Autodesk Inventor part; units mm, degrees
ref_plane "YZ Plane" through (0, 0, 0) normal (1, 0, 0) x (0, 1, 0)
ref_plane "XZ Plane" through (0, 0, 0) normal (0, 1, 0) x (-1, 0, 0)
ref_plane "XY Plane" through (0, 0, 0) normal (0, 0, 1) x (1, 0, 0)
sketch "Sketch1" plane through (0, 0, 0) normal (0, 1, 0) x (-1, 0, 0)
  circle A0 centre (0, 0) radius 25
  dimension "d0" = 50
extrude "Extrusion1" add sketch "Sketch1" against normal blind 15
sketch "Sketch3" plane through (0, 0, 0) normal (0, 1, 0) x (-1, 0, 0)
  circle A0 centre (0, 0) radius 15
  dimension "d3" = 30
extrude "Extrusion2" cut sketch "Sketch3" against normal through all
sketch "Sketch4" plane through (0, 0, 0) normal (0, 1, 0) x (-1, 0, 0)
  circle A0 centre (0, 0) radius 20
  dimension "d6" = 40
extrude "Extrusion3" cut sketch "Sketch4" against normal blind 12
properties part number "Седло для подшипника"
Geometry check sheet. Reference: the model listing, model coordinates, mm. Round coordinates to 2 decimals unless told otherwise and drop trailing zeros. Loops run counter-clockwise (first coordinate to the right, second up) from the corner with the lowest first, then second, coordinate; pieces in that order, holes last. Notation, with made-up numbers: (63, 37.25) - (102, 37.25) arc R17 ccw to (102, 47.25) - close; hole circle Ø11 at (51, -27). An arc over 180 degrees is marked (long way). Write each question's results on one line, items separated by ' | '. Start each with the question number.
Q1. Release check for a two-part mould opening along X. For faces 1 (the flat face through (-3, -12, 15)), 2 (the cylindrical face through (-23.846, -7.395, 7.509)), 3 (the flat face through (11, 0, 17)), 4 (the cylindrical face through (4.336, -5.916, -19.524)) record: +X half, -X half, draft (parallel to the pull), parting line (faces both ways), or undercut.
Q2. Cross-section at C-C on y = -10. Enter the section's corners in (x, z), and give its area (3 significant figures).
Q3. Cross-section at B-B on z = 0. Enter the section's corners in (x, y), and give its area (3 significant figures).
Q4. Cross-section at A-A on x = 0. Enter the section's corners in (y, z), and give its area (3 significant figures).
Q5. Thickness scan on line 1 (Z direction, x = 0, y = -13.3); line 2 (Z direction, x = 0, y = -3); line 3 (Y direction, x = -3.5, z = -19.5). Record the ranges inside material, lowest first. Write a range as [from, to].
Q6. Gauge pin test, flat ends, axial feed: P1, Ø2, axis at x = 17.5, z = -3, coming from the +Y side; P2, Ø1.5, axis at x = 1.5, y = -2.5, coming from the -Z side; P3, Ø1.5, axis at x = 10, y = -9, coming from the +Z side. Record the tip position at first contact, or that the pin passes through.
Q7. Cross-section at D-D on z = -18. Enter the section's corners in (x, y).
Answers below:
1) face 1: undercut | face 2: parting line | face 3: draft | face 4: undercut
2) outline: circle Ø50 at (0, 0); hole circle Ø40 at (0, 0) | area: 707 mm²
3) outline: (-25, -15) - (-15, -15) - (-15, -12) - (-20, -12) - (-20, 0) - (-25, 0) - close; (15, -15) - (25, -15) - (25, 0) - (20, 0) - (20, -12) - (15, -12) - close | area: 180 mm²
4) outline: (-15, -25) - (0, -25) - (0, -20) - (-12, -20) - (-12, -15) - (-15, -15) - close; (-15, 15) - (-12, 15) - (-12, 20) - (0, 20) - (0, 25) - (-15, 25) - close | area: 180 mm²
5) line 1: z = [-25, -15], [15, 25] | line 2: z = [-25, -20], [20, 25] | line 3: y = [-15, -12]
6) P1: stops at y = -12 | P2: stops at z = -24.99 | P3: stops at z = 23.23
7) outline: (-17.35, -15) - (17.35, -15) - (17.35, 0) - (8.72, 0) - (8.72, -12) - (-8.72, -12) - (-8.72, 0) - (-17.35, 0) - close
